```python
from build123d import *

# Parameters (mm, degrees)
SKETCH2_W           = 21.7
SKETCH2_H           = 4.7
SKETCH1_W           = 21.3
SKETCH1_H           = 4.7
SKETCH3_W           = 25.7
SKETCH3_H           = 6.7
BOSS_EXTRUDE1_DEPTH = 2
CHAMFER1_SIZE       = 0.7


with BuildPart() as part:
    # Sketch2 → Loft1 section 0
    with BuildSketch(Plane.XY.offset(2)):
        Rectangle(SKETCH2_W, SKETCH2_H)
    # Sketch1 → Loft1 section 1
    with BuildSketch(Plane.XY):
        Rectangle(SKETCH1_W, SKETCH1_H)
    loft()

    # Sketch3 → Boss-Extrude1 (add)
    with BuildSketch(Plane.XY.offset(2)):
        with Locations((0, -1)):
            Rectangle(SKETCH3_W, SKETCH3_H)
    extrude(amount=BOSS_EXTRUDE1_DEPTH)

    # Chamfer1
    chamfer1_edges = [part.edges().sort_by_distance(p)[0] for p in [
        (-12.85, -1, 4),
        (0, -4.35, 4),
        (12.85, -1, 4),
        (0, 2.35, 4),
    ]]
    chamfer(chamfer1_edges, length=CHAMFER1_SIZE)


solid = part.part
```
Geometry check sheet. Reference: the model listing, model coordinates, mm. A direction names the side the tool comes from. Give positions to 0.01 mm unless a question says otherwise; leave off trailing zeros. Loops run counter-clockwise (first coordinate to the right, second up) from the corner with the lowest first, then second, coordinate; pieces in that order, holes last. Notation, with made-up numbers: M -27.75,55.5 L 4.25,55.5 A25 ccw 4.25,69.5 Z; hole C 34,-35.75 d2. An arc over 180 degrees is marked long. Write item = value, one per line. Start each with the question number.
1. Section check B-B, the plane z = 3.75. Enter the section's corners in (x, y), plus the area to 3 significant figures.
2. Section check A-A, the plane y = -3. Enter the section's corners in (x, z), plus the area to 3 significant figures.
3. Thickness scan on probe 1 along Y at (x, z) = (-1.5, 0.8); probe 2 along Z at (x, y) = (-5.75, -3.5); probe 3 along X at (y, z) = (-1.25, 1.95) (3 decimals). Record the ranges inside material, lowest first.
4. Tool access check on faces 1 (the face through (0, -3, 2)), 2 (the face through (-10.75, 0.03, 0.99)). Record the directions out of +Z, -Z, +X, -X, +Y, -Y that give a thin tool (end or side, any length) a straight path to the whole face; none if there is none.
5. Section check C-C, the plane y = 1. Enter the section's corners in (x, z).
Values follow:
q1.outline = M -12.4,-3.9 L 12.4,-3.9 L 12.4,1.9 L -12.4,1.9 Z
q1.area = 144 mm^2
q2.outline = M -12.85,2 L 12.85,2 L 12.85,3.3 L 12.15,4 L -12.15,4 L -12.85,3.3 Z
q2.area = 50.9 mm^2
q3.probe_1 = -2.35 to 2.35
q3.probe_2 = 2 to 4
q3.probe_3 = -10.845 to 10.845
q4.face_1 = -Z, -Y
q4.face_2 = -Z, -X, +Y, -Y
q5.outline = M -12.85,2 L -10.85,2 L -10.65,0 L 10.65,0 L 10.85,2 L 12.85,2 L 12.85,3.3 L 12.15,4 L -12.15,4 L -12.85,3.3 Z
